from build123d import *

# Parameters (mm, degrees)
SKETCH1_W           = 28
SKETCH1_H           = 46
BOSS_EXTRUDE1_DEPTH = 10
SKETCH2_W           = 20
SKETCH2_H           = 6
CUT_EXTRUDE1_DEPTH  = 50.112116631
FILLET3_R           = 1


with BuildPart() as part:
    # Sketch1 → Boss-Extrude1 (new body)
    with BuildSketch(Plane(origin=(0, 0, 0), x_dir=(1, 0, 0), z_dir=(0, 1, 0))):
        Rectangle(SKETCH1_W, SKETCH1_H)
    extrude(amount=BOSS_EXTRUDE1_DEPTH)

    # Sketch2 → Cut-Extrude1 (cut, through all)
    with BuildSketch(Plane.XY.offset(23)):
        with Locations((0, 3)):
            Rectangle(SKETCH2_W, SKETCH2_H)
    extrude(amount=-CUT_EXTRUDE1_DEPTH, mode=Mode.SUBTRACT)

    # Sketch3 → Cut-Revolve1 (revolve, cut)
    with BuildSketch(Plane.XY, mode=Mode.PRIVATE) as cut_revolve1_sk:
        with BuildLine():
            Line((5.375181252, 8.187051569), (4.715321987, 10))
            Line((4.715321987, 10), (7.754678013, 10))
            Line((7.754678013, 10), (7.094818748, 8.187051569))
            ThreePointArc((7.094818748, 8.187051569), (6.235, 7.585), (5.375181252, 8.187051569))
        make_face()
    revolve(cut_revolve1_sk.sketch.rotate(Axis((0, -1000.11801834, 0), (0, 1, 0)), 90), axis=Axis((0, -1000.11801834, 0), (0, 1, 0)), mode=Mode.SUBTRACT)

    # Fillet3
    fillet3_edges = [part.edges().sort_by_distance(p)[0] for p in [
        (0, 10, 7.754678013),
        (0, 10, 4.715321987),
    ]]
    fillet(fillet3_edges, radius=FILLET3_R)


solid = part.part
Here's how the part is built. I have some questions about the finished solid (model axes, mm). A direction names the side the tool comes from. Give positions to 0.01 mm unless a question says otherwise; leave off trailing zeros. Write each loop counter-clockwise with the first axis right and the second up, starting at its lowest first coordinate (ties: lowest second). Pieces come first, ordered by that corner, then holes. Notation, with made-up numbers: (8, 66.5) -> (25, 66.5) arc R21 ccw to (25, 95.5) -> close; hole circle Ø4 at (33.5, -10). An arc over 180 degrees is marked (long way). Use one line per item in the form item = value. Start each with the question number.
1. Imagine slicing it at A-A on y = 1.75. List the corners of the cut face in (x, z) for me.
2. If I drill on L1, parallel to X at y = 3, z = -11.5; L2, parallel to Z at x = 2.5, y = 9; L3, parallel to X at y = 9.5, z = 1, over which ranges is the centre line in solid material (lowest first)?
3. Imagine slicing it at B-B on z = 0. List the corners of the cut face in (x, y) for me (3 decimals).
4. Imagine slicing it at D-D on z = 12. List the corners of the cut face in (x, y) for me, plus the area to 3 significant figures.
5. Imagine slicing it at C-C on x = 0. List the corners of the cut face in (y, z) for me (3 decimals), plus the area to 3 significant figures.
6. Will these pins go through, and if not, where does the flat tip stop? pin 1 Ø10 at (x, z) = (4.5, 0.5) entering from -Y; pin 2 Ø10 at (x, z) = (-7, -5.5) entering from -Y.
7. On a 3-axis mill with a long thin cutter (end or side, diameter ignored), from which of +Z, -Z, +X, -X, +Y, -Y can I reach the whole of each face in a straight line? I mean faces 1 (the face through (-12, 0, 0)), 2 (the face through (-10, 3, 0)). Say none if no direction works.
Entries:
q1.outline = (-14, -23) -> (-10, -23) -> (-10, 23) -> (-14, 23) -> close; (10, -23) -> (14, -23) -> (14, 23) -> (10, 23) -> close
q2.L1 = -14 to -10, 10 to 14
q2.L2 = -23 to -6.96, -4.42 to 4.42, 6.96 to 23
q2.L3 = -14 to -7.52, -4.78 to 4.78, 7.52 to 14
q3.outline = (-14, 0) -> (-10, 0) -> (-10, 6) -> (10, 6) -> (10, 0) -> (14, 0) -> (14, 10) -> (8.455, 10) arc R1 ccw to (7.515, 9.342) -> (7.095, 8.187) arc R0.915 cw to (5.375, 8.187) -> (4.955, 9.342) arc R1 ccw to (4.015, 10) -> (-4.015, 10) arc R1 ccw to (-4.955, 9.342) -> (-5.375, 8.187) arc R0.915 cw to (-7.095, 8.187) -> (-7.515, 9.342) arc R1 ccw to (-8.455, 10) -> (-14, 10) -> close
q4.outline = (-14, 0) -> (-10, 0) -> (-10, 6) -> (10, 6) -> (10, 0) -> (14, 0) -> (14, 10) -> (-14, 10) -> close
q4.area = 160 mm²
q5.outline = (6, -23) -> (10, -23) -> (10, -8.455) arc R1 ccw to (9.342, -7.515) -> (8.187, -7.095) arc R0.915 cw to (8.187, -5.375) -> (9.342, -4.955) arc R1 ccw to (10, -4.015) -> (10, 4.015) arc R1 ccw to (9.342, 4.955) -> (8.187, 5.375) arc R0.915 cw to (8.187, 7.095) -> (9.342, 7.515) arc R1 ccw to (10, 8.455) -> (10, 23) -> (6, 23) -> close
q5.area = 174 mm²
q6.pin_1 = 6
q6.pin_2 = 0
q7.face_1 = +Z, -Z, +X, -X, -Y
q7.face_2 = +Z, -Z, -Y
